```python
from build123d import *

# Parameters (mm, degrees)
F1_DEPTH = 30
F2_R     = 7.5
F3_DEPTH = 30
F5_DEPTH = 21
F6_W     = 27
F6_H     = 7
F7_DEPTH = 21
F9_DEPTH = 25


with BuildPart() as f1:
    # F0 (on Top) → F1 (new body)
    with BuildSketch(Plane.XY):
        with BuildLine():
            Line((21, 15), (-15, 15))
            ThreePointArc((-15, 15), (-30, 0), (-15, -15))
            Line((-15, -15), (21, -15))
            Line((21, -15), (30, -6))
            Line((30, -6), (30, 6))
            Line((30, 6), (21, 15))
        make_face()
    extrude(amount=F1_DEPTH)

    # F2 (on face) → F3 (cut)
    with BuildSketch(Plane.XY.offset(30)):
        with Locations((-15, 0)):
            Circle(F2_R)
    extrude(amount=-F3_DEPTH, mode=Mode.SUBTRACT)

    # F4 (on face) → F5 (cut)
    with BuildSketch(Plane(origin=(0, 0, 0), x_dir=(1, 0, 0), z_dir=(0, 0, -1))):
        Polygon((21, 15), (3, 15), (3, -15), (21, -15), (30, -6), (30, 6), align=None)
    extrude(amount=-F5_DEPTH, mode=Mode.SUBTRACT)

    # F6 (on face) → F7 (join)
    with BuildSketch(Plane(origin=(0, 0, 21), x_dir=(1, 0, 0), z_dir=(0, 0, -1))):
        with Locations((16.5, 0)):
            Rectangle(F6_W, F6_H)
    extrude(amount=F7_DEPTH)

    # F8 (on face) → F9 (cut)
    with BuildSketch(Plane(origin=(0, 3.5, 0), x_dir=(-1, 0, 0), z_dir=(0, 1, 0))):
        Polygon((-30, 0), (-3, 0), (-30, 21), align=None)
    extrude(amount=-F9_DEPTH, mode=Mode.SUBTRACT)


solid = f1.part
```
Read the model definition and answer for the solid it produces. Units are mm, in the model's axes. A direction names the side the tool comes from. Coordinates: 2 decimals unless noted, no trailing zeros. Write each loop counter-clockwise with the first axis right and the second up, starting at its lowest first coordinate (ties: lowest second). Pieces come first, ordered by that corner, then holes. Notation, with made-up numbers: (48.5, 17) -> (99.5, 17) arc R25 ccw to (99.5, 41) -> close; hole circle Ø3 at (46, 47). An arc over 180 degrees is marked (long way). Answer as a JSON object with one key per item and string values.
Q1. Flat-ended cylindrical pins translate along their axes: pin 1 Ø1.5 at (y, z) = (1, 6.5) entering from -X; pin 2 Ø9 at (y, z) = (10.5, 12) entering from +X; pin 3 Ø3.5 at (x, y) = (15, -8.5) entering from -Z. Find the tip coordinate at first contact, or state that the pin passes through.
The answers:
{"pin 1": "stops at x = -30", "pin 2": "stops at x = 3", "pin 3": "stops at z = 21"}
Q2. A tool of negligible diameter and unlimited length cuts with its end or side. For faces 1 (the flat face through (-1, -15, 18)), 2 (the flat face through (16, -9, 21)), 3 (the flat face through (16, 9, 21)), from which of +Z, -Z, +X, -X, +Y, -Y can it reach the whole face along a straight path? Write none if from no direction.
The answers:
{"face 1": "+Z, -Z, +X, -X, -Y", "face 2": "-Z, +X, -Y", "face 3": "-Z, +X, +Y"}
Q3. The part is cut by section D-D on z = 9.75. Give the vertices of the cut face in (x, y), then the cut area to 3 significant figures.
The answers:
{"outline": "(-15, -15) -> (3, -15) -> (3, -3.5) -> (15.54, -3.5) -> (15.54, 3.5) -> (3, 3.5) -> (3, 15) -> (-15, 15) arc R15 ccw to start; hole circle Ø15 at (-15, 0)", "area": "804 mm2"}
Q4. Determine the mould class of faces 4 (the flat face through (-6, 0, 0)), 5 (the cylindrical face through (-22.493, 0.33, 15.21)), 6 (the flat face through (3, 9, 10)) for opening direction X: pulls with the +X half, pulls with the -X half, needs draft (parallel to the pull), parting line crosses it, or undercut.
The answers:
{"face 4": "needs draft", "face 5": "undercut", "face 6": "pulls with the +X half"}
Q5. The part is cut by section A-A on y = 0. Give the vertices of the cut face in (x, z), then the cut area to 3 significant figures.
The answers:
{"outline": "(-30, 0) -> (-22.5, 0) -> (-22.5, 30) -> (-30, 30) -> close; (-7.5, 0) -> (3, 0) -> (30, 21) -> (30, 30) -> (-7.5, 30) -> close", "area": "1,070 mm2"}
Q6. The part is cut by section B-B on z = 23.5. Give the vertices of the cut face in (x, y), then the cut area to 3 significant figures.
The answers:
{"outline": "(-15, -15) -> (21, -15) -> (30, -6) -> (30, 6) -> (21, 15) -> (-15, 15) arc R15 ccw to start; hole circle Ø15 at (-15, 0)", "area": "1,450 mm2"}
Q7. The part is cut by section C-C on x = 14. Give the vertices of the cut face in (y, z).
The answers:
{"outline": "(-15, 21) -> (-3.5, 21) -> (-3.5, 8.56) -> (3.5, 8.56) -> (3.5, 21) -> (15, 21) -> (15, 30) -> (-15, 30) -> close"}
Q8. Consider line 1 (Y direction, x = -15, z = 15.5); line 2 (Z direction, x = 25.5, y = -4); line 3 (X direction, y = -2.5, z = 7.25). Determine where each line is inside the solid, lowest interval first. Write a range as [from, to].
The answers:
{"line 1": "y = [-15, -7.5], [7.5, 15]", "line 2": "z = [21, 30]", "line 3": "x = [-29.79, -22.07], [-7.93, 12.32]"}
